from build123d import *

# Parameters (mm, degrees)
F1_R     = 4.25
F2_DEPTH = 20
F0_R     = 4.25
F4_DEPTH = 20
F3_R     = 2.5
F5_DEPTH = 40
F6_R     = 2.5
F7_DEPTH = 20


with BuildPart() as f2:
    # F1 (on Front) → F2 (new body, symmetric)
    with BuildSketch(Plane.XZ):
        Circle(F1_R)
    extrude(amount=F2_DEPTH, both=True)

    # F0 (on Top) → F4 (join)
    with BuildSketch(Plane.XY):
        Circle(F0_R)
    extrude(amount=F4_DEPTH)

    # F3 (on face) → F5 (cut)
    with BuildSketch(Plane.XZ.offset(20)):
        Circle(F3_R)
    extrude(amount=-F5_DEPTH, mode=Mode.SUBTRACT)

    # F6 (on face) → F7 (cut)
    with BuildSketch(Plane.XY.offset(20)):
        Circle(F6_R)
    extrude(amount=-F7_DEPTH, mode=Mode.SUBTRACT)


solid = f2.part
The model under review builds one solid part; all positions refer to its coordinate system, in mm. A direction names the side the tool comes from. Give positions to 0.01 mm unless a question says otherwise; leave off trailing zeros. Order: outer loops, then holes, each group sorted by start corner. A loop starts at its lowest first (then second) coordinate and runs counter-clockwise, first axis right, second up. Notation, with made-up numbers: M -14,-4 L 29,-4 A10 cw 29,10 Z; hole C -0.75,54 d8. An arc over 180 degrees is marked long. Use one line per item in the form item = value. Start each with the question number.
Item 1: We need section D-D on x = 3.25. Give the boundary of the cut face in (y, z), plus the area to 3 significant figures.
Item 2: We need section A-A on x = -2. Give the boundary of the cut face in (y, z), plus the area to 3 significant figures.
Item 3: We need section C-C on y = 0. Give the boundary of the cut face in (x, z).
Item 4: Insertion check: pin 1 Ø1.5 at (x, z) = (2, 9) entering from +Y. The pin has a flat end and moves straight along its axis. Give the tip position at first contact, or say it passes through.
Item 5: For faces 4 (the flat face through (2, -20, -2)), 5 (the cylindrical face through (2.385, 0.751, 10.14)), list the 3-axis set-ups (+Z, -Z, +X, -X, +Y, -Y) from which the entire face can be reached by the end or side of a thin tool; tool diameter is ignored.
Item 6: The part is to be moulded in two halves that separate along X. For faces 1 (the flat face through (2, 20, -2)), 2 (the cylindrical face through (-0.92, -0.28, -4.15)), 3 (the cylindrical face through (-0.54, -0.28, -2.44)), say which applies: pulls with the +X half, pulls with the -X half, needs draft (parallel to the pull), parting line crosses it, or undercut.
Item 7: To check wall thickness, follow line 1 along Y through (x, z) = (0, 7); line 2 along Z through (x, y) = (0, -3). State the ranges of each line that lie inside material, in increasing order. Write a range as from..to.
Item 8: We need section B-B on z = -0.75. Give the boundary of the cut face in (x, y).
Completed:
q1.outline = M -20,-2.74 L 20,-2.74 L 20,2.74 L 2.74,2.74 L 2.74,20 L -2.74,20 L -2.74,2.74 L -20,2.74 Z
q1.area = 314 mm²
q2.outline = M -20,-3.75 L 20,-3.75 L 20,-1.5 L -20,-1.5 Z; M -20,1.5 L -1.5,1.5 L -1.5,20 L -3.75,20 L -3.75,3.75 L -20,3.75 Z; M 1.5,1.5 L 20,1.5 L 20,3.75 L 3.75,3.75 L 3.75,20 L 1.5,20 Z
q2.area = 246 mm²
q3.outline = M -4.25,0 A4.25 ccw 4.25,0 L 4.25,20 L 2.5,20 L 2.5,0 A2.5 cw -2.5,0 L -2.5,20 L -4.25,20 Z
q4.pin_1 = 4.06
q5.face_4 = +Z, -Z, +X, -X, -Y
q5.face_5 = +Z
q6.face_1 = needs draft
q6.face_2 = parting line crosses it
q6.face_3 = undercut
q7.line_1 = -4.25..-2.5, 2.5..4.25
q7.line_2 = -4.25..-2.5, 2.5..20
q8.outline = M -4.18,-20 L -2.38,-20 L -2.38,20 L -4.18,20 Z; M 2.38,-20 L 4.18,-20 L 4.18,20 L 2.38,20 Z
